```python
from build123d import *

# Parameters (mm, degrees)
F0_W     = 58
F0_H     = 76
F0_W_2   = 42
F0_H_2   = 60
F1_DEPTH = 25
F2_R     = 9.625
F3_DEPTH = 58
F4_R     = 4.1
F5_DEPTH = 76
F6_R     = 9.625
F6_R_2   = 7.625
F7_DEPTH = 1
F8_R     = 9.625
F8_R_2   = 7.625
F9_DEPTH = 1


with BuildPart() as f1:
    # F0 (on Top) → F1 (new body)
    with BuildSketch(Plane.XY):
        Rectangle(F0_W, F0_H)
        Rectangle(F0_W_2, F0_H_2, mode=Mode.SUBTRACT)
    extrude(amount=F1_DEPTH)

    # F2 (on face) → F3 (cut, through all)
    with BuildSketch(Plane(origin=(-29, 0, 0), x_dir=(0, -1, 0), z_dir=(-1, 0, 0))):
        with Locations((0, 12.5)):
            Circle(F2_R)
    extrude(amount=-F3_DEPTH, mode=Mode.SUBTRACT)

    # F4 (on face) → F5 (cut, through all)
    with BuildSketch(Plane.XZ.offset(38)):
        with Locations((0, 12.5)):
            Circle(F4_R)
    extrude(amount=-F5_DEPTH, mode=Mode.SUBTRACT)

    # F6 (on face) → F7 (join)
    with BuildSketch(Plane(origin=(21, 0, 0), x_dir=(0, -1, 0), z_dir=(-1, 0, 0))):
        with Locations((0, 12.5)):
            Circle(F6_R)
        with Locations((0, 12.5)):
            Circle(F6_R_2, mode=Mode.SUBTRACT)
    extrude(amount=-F7_DEPTH)

    # F8 (on face) → F9 (join)
    with BuildSketch(Plane.YZ.offset(-21)):
        with Locations((0, 12.5)):
            Circle(F8_R)
        with Locations((0, 12.5)):
            Circle(F8_R_2, mode=Mode.SUBTRACT)
    extrude(amount=-F9_DEPTH)


solid = f1.part
```
Check sheet for the modelled part. Datum: model origin and axes. Units: mm. A direction names the side the tool comes from. Round coordinates to 2 decimals unless told otherwise and drop trailing zeros. Order: outer loops, then holes, each group sorted by start corner. A loop starts at its lowest first (then second) coordinate and runs counter-clockwise, first axis right, second up. Notation, with made-up numbers: (83, 34.5) - (112, 34.5) arc R15 cw to (112, 45.5) - close; hole circle Ø3 at (88.5, 27). An arc over 180 degrees is marked (long way). Write item = value, one per line.
Q1. Thickness scan on line 1 along Y through (x, z) = (15.5, 6.5); line 2 along X through (y, z) = (-15.5, 10.5); line 3 along Z through (x, y) = (-26, 0) (3 decimals). Record the ranges inside material, lowest first.
Computed:
line_1 = -38 to -30, 30 to 38
line_2 = -29 to -21, 21 to 29
line_3 = 0 to 2.875, 22.125 to 25
Q2. Draft check along X on faces 4 (the face through (-25.549, 7.638, 6.643)), 5 (the face through (-0.9, -34.1, 8.5)), 6 (the face through (22, 6, 18)), 7 (the face through (-22, -6, 18)). Enter one of: pulls with the +X half, pulls with the -X half, needs draft (parallel to the pull), parting line crosses it, or undercut.
Computed:
face_4 = needs draft
face_5 = undercut
face_6 = pulls with the +X half
face_7 = pulls with the -X half
Q3. Tool access check on faces 1 (the face through (21, 0, 21)), 2 (the face through (-21.493, -5.62, 17.653)), 3 (the face through (25.451, 7.638, 6.643)). Record the directions out of +Z, -Z, +X, -X, +Y, -Y that give a thin tool (end or side, any length) a straight path to the whole face; none if there is none.
Computed:
face_1 = +Z, -Z
face_2 = +X, -X
face_3 = +X
Q4. Go/stop test with flat-tipped pins: pin 1 (9 mm diameter, centred on y = 0, z = 12.5, fed in from +X); pin 2 (6 mm diameter, centred on y = 2, z = 17, fed in from -X); pin 3 (4 mm diameter, centred on y = 2, z = 6, fed in from +X). Record where each tip stops, or that it passes through.
Computed:
pin_1 = through
pin_2 = -22
pin_3 = 22
Q5. Section check D-D (x = 0). Record the boundary of the cut face in (y, z), and give its area (3 significant figures).
Computed:
outline = (-38, 0) - (-30, 0) - (-30, 8.4) - (-38, 8.4) - close; (-38, 16.6) - (-30, 16.6) - (-30, 25) - (-38, 25) - close; (30, 0) - (38, 0) - (38, 8.4) - (30, 8.4) - close; (30, 16.6) - (38, 16.6) - (38, 25) - (30, 25) - close
area = 269 mm^2
Q6. Section check B-B (z = 12.5). State how many separate pieces and enclosed holes the cut face has, and give its area (3 significant figures).
Computed:
separate_pieces = 4
enclosed_holes = 0
area = 1,460 mm^2
Q7. Section check A-A (y = 0). Record the boundary of the cut face in (x, z) (3 decimals).
Computed:
outline = (-29, 0) - (-21, 0) - (-21, 4.875) - (-22, 4.875) - (-22, 2.875) - (-29, 2.875) - close; (-29, 22.125) - (-22, 22.125) - (-22, 20.125) - (-21, 20.125) - (-21, 25) - (-29, 25) - close; (21, 0) - (29, 0) - (29, 2.875) - (22, 2.875) - (22, 4.875) - (21, 4.875) - close; (21, 20.125) - (22, 20.125) - (22, 22.125) - (29, 22.125) - (29, 25) - (21, 25) - close
Q8. Section check C-C (y = -14.5). Record the boundary of the cut face in (x, z).
Computed:
outline = (-29, 0) - (-21, 0) - (-21, 25) - (-29, 25) - close; (21, 0) - (29, 0) - (29, 25) - (21, 25) - close
